```python
from build123d import *

# Parameters (mm, degrees)
F3_DEPTH = 5
F4_D     = 2
F5_D     = 2


# Not quite as in the source:
# - a feature names something its author has since deleted; it is built from what else it names


with BuildPart() as f3:
    # F2 (on Front) → F3 (new body)
    with BuildSketch(Plane.XZ):
        with BuildLine():
            ThreePointArc((12.9616053321, -5), (16.4971392381, -3.5355339059), (17.9616053321, 0))
            ThreePointArc((17.9616053321, 0), (16.4971392381, 3.5355339059), (12.9616053321, 5))
            ThreePointArc((12.9616053321, 5), (7.9616053321, 0), (12.9616053321, -5))
        make_face()
        with BuildLine():
            ThreePointArc((12.9616053321, -5), (7.9616053321, 0), (12.9616053321, 5))
            Line((12.9616053321, 5), (-17.8376678377, 5))
            ThreePointArc((-17.8376678377, 5), (-14.3021339318, 3.5355339059), (-12.8376678377, 0))
            ThreePointArc((-12.8376678377, 0), (-14.3021339318, -3.5355339059), (-17.8376678377, -5))
            Line((-17.8376678377, -5), (12.9616053321, -5))
        make_face()
        with BuildLine():
            ThreePointArc((-12.8376678377, 0), (-14.3021339318, 3.5355339059), (-17.8376678377, 5))
            ThreePointArc((-17.8376678377, 5), (-22.8376678377, 0), (-17.8376678377, -5))
            ThreePointArc((-17.8376678377, -5), (-14.3021339318, -3.5355339059), (-12.8376678377, 0))
        make_face()
    extrude(amount=F3_DEPTH)

    # F4 (through all)
    with Locations(Plane(origin=(0, 0, 0), x_dir=(1, 0, 0), z_dir=(0, 1, 0))):
        with Locations((12.9616053321, 0)):
            Hole(F4_D / 2)

    # F5 (through all)
    with Locations(Plane(origin=(0, 0, 0), x_dir=(1, 0, 0), z_dir=(0, 1, 0))):
        with Locations((-17.8376678377, 0)):
            Hole(F5_D / 2)


solid = f3.part
```
Part model, mm, in its own coordinate system. Round coordinates to 2 decimals unless told otherwise and drop trailing zeros. Write each loop counter-clockwise with the first axis right and the second up, starting at its lowest first coordinate (ties: lowest second). Pieces come first, ordered by that corner, then holes. Notation, with made-up numbers: M 75,46 L 120,46 A26 ccw 120,74 Z; hole C 25,59.25 d4. An arc over 180 degrees is marked long. One line per question, with ' | ' between items.
(1) Saw through at C-C on x = -19.5. Write the cut outline in (y, z).
Answer key:
outline: M -5,-4.72 L 0,-4.72 L 0,4.72 L -5,4.72 Z
(2) Saw through at B-B on z = 2.5. Write the cut outline in (x, y), then the cut area to 3 significant figures.
Answer key:
outline: M -22.17,-5 L 17.29,-5 L 17.29,0 L -22.17,0 Z | area: 197 mm^2
(3) Pin check, flat tips, straight feed: pin 1 (1 mm diameter, centred on y = -1.5, z = -3.5, fed in from +X); pin 2 (1.5 mm diameter, centred on y = -1.5, z = 4, fed in from +X). Stop position of each tip, or through.
Answer key:
pin 1: stops at x = 16.96 | pin 2: stops at x = 16.76
(4) Two-plate mould, pull along X, no slides. Class faces 1 (the face through (-22.836, -2.465, 0.11)), 2 (the face through (13.96, -2.54, -0.04)), 3 (the face through (-3, -2, -5)): released by +X, released by -X, zero draft, split by the parting line, or undercut.
Answer key:
face 1: released by -X | face 2: undercut | face 3: zero draft
(5) Probe line 1 along Z through (x, y) = (-17, -3.25); line 2 along Z through (x, y) = (12.5, -2.75); line 3 along X through (y, z) = (-0.9, 2.25). List the from-to ranges inside material, lowest first.
Answer key:
line 1: z = -5 to -0.55, 0.55 to 5 | line 2: z = -5 to -0.89, 0.89 to 5 | line 3: x = -22.3 to 17.43
(6) Saw through at A-A on y = -2.4. Write the cut outline in (x, z).
Answer key:
outline: M -17.84,-5 L 12.96,-5 A5 ccw 12.96,5 L -17.84,5 A5 ccw Z; hole C -17.84,0 d2; hole C 12.96,0 d2
